Could you check a few things on this model? Use its own coordinates, in mm. A direction names the side the tool comes from. Round coordinates to 2 decimals unless told otherwise and drop trailing zeros. Loops run counter-clockwise (first coordinate to the right, second up) from the corner with the lowest first, then second, coordinate; pieces in that order, holes last. Notation, with made-up numbers: (-5.5, -38) -> (7.5, -38) arc R12 ccw to (7.5, -30) -> close; hole circle Ø1 at (-35.5, -35.5). An arc over 180 degrees is marked (long way). One line per item, written item: value.
```python
from build123d import *

# Parameters (mm, degrees)
SKETCH_1_R      = 2.5
EXTRUDE_1_DEPTH = 4
FILLET_1_R      = 5
SKETCH_2_R      = 2.5
EXTRUDE_2_DEPTH = 10


with BuildPart() as part:
    # ｽｹｯﾁ1 → ﾎﾞｽ - 押し出し1 (new body)
    with BuildSketch(Plane.XY):
        Polygon((0, 15), (0, 0), (4, 0), (4, -6), (8.110763801, -6), (24, -2.18322685), (24, 8.312378031), (4, 22), (4, 15), align=None)
        with Locations((14, 3)):
            Circle(SKETCH_1_R, mode=Mode.SUBTRACT)
    extrude(amount=EXTRUDE_1_DEPTH)

    # ﾌｨﾚｯﾄ1
    fillet_1_edges = [part.edges().sort_by_distance(p)[0] for p in [
        (24, -2.18322685, 2),
        (24, 8.312378031, 2),
    ]]
    fillet(fillet_1_edges, radius=FILLET_1_R)

    # ｽｹｯﾁ2 → ﾎﾞｽ - 押し出し2 (add)
    with BuildSketch(Plane.XY.offset(4)):
        with BuildLine():
            Line((4, 0), (4, -6))
            Line((4, -6), (8.110763801, -6))
            Line((8.110763801, -6), (20.167835798, -3.103755769))
            ThreePointArc((20.167835798, -3.103755769), (22.926778514, -1.337276232), (24, 1.757947589))
            Line((24, 1.757947589), (24, 5.675452184))
            ThreePointArc((24, 5.675452184), (23.422640317, 8.007887097), (21.823898951, 9.801660457))
            Line((21.823898951, 9.801660457), (12.911949475, 15.900830229))
            Line((12.911949475, 15.900830229), (4, 0))
        make_face()
        with Locations((14, 3)):
            Circle(SKETCH_2_R, mode=Mode.SUBTRACT)
    extrude(amount=EXTRUDE_2_DEPTH)


solid = part.part
```
Item 1: If we section it at D-D on y = -0.5: List the corners of the cut face in (x, z) for me, plus the area to 3 significant figures.
Output:
outline: (4, 0) -> (23.46, 0) -> (23.46, 14) -> (4, 14) -> close
area: 272 mm²
Item 2: If we section it at C-C on y = 3: List the corners of the cut face in (x, z) for me.
Output:
outline: (0, 0) -> (11.5, 0) -> (11.5, 14) -> (5.68, 14) -> (5.68, 4) -> (0, 4) -> close; (16.5, 0) -> (24, 0) -> (24, 14) -> (16.5, 14) -> close
Item 3: Will these pins go through, and if not, where does the flat tip stop? pin 1 Ø4.5 at (x, z) = (1.5, 3) entering from -Y; pin 2 Ø5 at (y, z) = (-4, 8) entering from -X; pin 3 Ø4 at (x, z) = (19.5, 10.5) entering from +Y.
Output:
pin 1: stops at y = 0
pin 2: stops at x = 4
pin 3: stops at y = 12.76
Item 4: For faces 1 (the face through (8.518, 8.062, 8.93)), 2 (the face through (4, -3, 7)), 3 (the face through (2, 15, 2)), which set-ups out of +Z, -Z, +X, -X, +Y, -Y let a thin tool reach every point of the face, with its end or its side?
Output:
face 1: +Z, -X, +Y
face 2: +Z, -Z, -X, -Y
face 3: +Z, -Z, -X, +Y
Item 5: If we section it at B-B on x = 14: List the corners of the cut face in (y, z) for me.
Output:
outline: (-4.59, 0) -> (0.5, 0) -> (0.5, 14) -> (-4.59, 14) -> close; (5.5, 0) -> (15.16, 0) -> (15.16, 14) -> (5.5, 14) -> close
Item 6: If we section it at A-A on z = 12: List the corners of the cut face in (x, y) for me.
Output:
outline: (4, -6) -> (8.11, -6) -> (20.17, -3.1) arc R5 ccw to (24, 1.76) -> (24, 5.68) arc R5 ccw to (21.82, 9.8) -> (12.91, 15.9) -> (4, 0) -> close; hole circle Ø5 at (14, 3)
Item 7: If we mould it in two halves opening along X, with no side actions, what happens to faces 4 (the face through (4, 19, 2)), 5 (the face through (11.5, 3.1, 6.9)), 6 (the face through (5, 11, 4))? For each: released by +X, released by -X, zero draft, split by the parting line, or undercut.
Output:
face 4: released by -X
face 5: undercut
face 6: zero draft
Item 8: I need wall thicknesses on line 1 (Z direction, x = 6.75, y = 7.5); line 2 (Y direction, x = 13, z = 6); line 3 (Y direction, x = 14, z = 10.5). Which ranges of each line are inside material? Lowest first, please. Write a range as from..to.
Output:
line 1: z = 0..4
line 2: y = -4.83..0.71, 5.29..15.84
line 3: y = -4.59..0.5, 5.5..15.16
